Read the model definition and answer for the solid it produces. Units are mm, in the model's axes. A direction names the side the tool comes from. Coordinates: 2 decimals unless noted, no trailing zeros. Write each loop counter-clockwise with the first axis right and the second up, starting at its lowest first coordinate (ties: lowest second). Pieces come first, ordered by that corner, then holes.
Item 1: Straight lines are drawn through the part: probe 1 along X at (y, z) = (-6, -6.5); probe 2 along Z at (x, y) = (8.5, 3); probe 3 along X at (y, z) = (-8, -4). For each, find the intervals that lie inside material, in ascending order.
Item 2: Section A-A (z = -1.75) is taken. Give the vertices of the cut face in (x, y), then the cut area to 3 significant figures.
Item 3: Section B-B (x = 24.5) is taken. Give the vertices of the cut face in (y, z), then the cut area to 3 significant figures.
Item 4: Each of these flat-tipped pins is pushed along its axis until it touches: P1, Ø1, axis at y = 1.5, z = -5, coming from the -X side; P2, Ø1.5, axis at x = 15, y = 3, coming from the -Z side; P3, Ø2, axis at y = -1.5, z = -6, coming from the -X side. Where does it stop, or does it pass through?
Item 5: A tool of negligible diameter and unlimited length cuts with its end or side. For faces 4 (the face through (53, 9, 0)), 5 (the face through (84.524, 2.772, 5.986)), 6 (the face through (107, 0, -6)), from which of +Z, -Z, +X, -X, +Y, -Y can it reach the whole face along a straight path? Write none if from no direction.
Item 6: Determine the mould class of faces 1 (the face through (33, -9, 0)), 2 (the face through (84.108, 0.815, -0.098)), 3 (the face through (-9, 0, 0)) for opening direction X: released by +X, released by -X, zero draft, split by the parting line, or undercut.
Item 7: Section C-C (x = 81) is taken. Give the vertices of the cut face in (y, z).
from build123d import *
from build123d.topology import SkipClean

# Parameters (mm, degrees)
BOSS_EXTRUDE1_DEPTH = 5
BOSS_EXTRUDE2_START = -12
BOSS_EXTRUDE2_DEPTH = 14


with BuildPart() as part:
    # Sketch1 → Boss-Extrude1 (new, symmetric)
    with SkipClean():  # the faces are left unmerged after this step: merging them gives an invalid solid
        with BuildSketch(Plane.XY):
            with BuildLine():
                ThreePointArc((9, 0), (6.363961031, -6.363961031), (0, -9))
                Line((0, -9), (66.272706331, -9))
                ThreePointArc((66.272706331, -9), (68.43776984, -7.75), (68.43776984, -5.25))
                ThreePointArc((68.43776984, -5.25), (67.583242863, 0.670186682), (73.015870906, 3.173260641))
                Line((73.015870906, 3.173260641), (95.515870906, -1.609261996))
                ThreePointArc((95.515870906, -1.609261996), (97.934586459, -2.888858783), (99.317541634, -5.25))
                ThreePointArc((99.317541634, -5.25), (104.158770817, -9), (109, -5.25))
                Line((109, -5.25), (109, 5))
                ThreePointArc((109, 5), (107.828427125, 7.828427125), (105, 9))
                Line((105, 9), (0, 9))
                ThreePointArc((0, 9), (6.363961031, 6.363961031), (9, 0))
            make_face()
            with BuildLine():
                ThreePointArc((-9, 0), (-6.363961031, -6.363961031), (0, -9))
                ThreePointArc((0, -9), (6.363961031, -6.363961031), (9, 0))
                Line((9, 0), (4.75, 0))
                ThreePointArc((4.75, 0), (0, -4.75), (-4.75, 0))
                Line((-4.75, 0), (-9, 0))
            make_face()
            with BuildLine():
                ThreePointArc((0, 9), (-6.363961031, 6.363961031), (-9, 0))
                Line((-9, 0), (-4.75, 0))
                ThreePointArc((-4.75, 0), (0, 4.75), (4.75, 0))
                Line((4.75, 0), (9, 0))
                ThreePointArc((9, 0), (6.363961031, 6.363961031), (0, 9))
            make_face()
            with BuildLine():
                ThreePointArc((-9, 0), (-6.363961031, -6.363961031), (0, -9))
                ThreePointArc((0, -9), (6.363961031, -6.363961031), (9, 0))
                Line((9, 0), (4.75, 0))
                ThreePointArc((4.75, 0), (0, -4.75), (-4.75, 0))
                Line((-4.75, 0), (-9, 0))
            make_face()
            with BuildLine():
                ThreePointArc((0, 9), (-6.363961031, 6.363961031), (-9, 0))
                Line((-9, 0), (-4.75, 0))
                ThreePointArc((-4.75, 0), (0, 4.75), (4.75, 0))
                Line((4.75, 0), (9, 0))
                ThreePointArc((9, 0), (6.363961031, 6.363961031), (0, 9))
            make_face()
        extrude(amount=BOSS_EXTRUDE1_DEPTH, both=True)

    # Sketch2 → Boss-Extrude2 (add)
    with SkipClean():  # the faces are left unmerged after this step: merging them gives an invalid solid
        with BuildSketch(Plane.XY.offset(5).offset(BOSS_EXTRUDE2_START)):
            with BuildLine():
                Line((105, 9), (0, 9))
                ThreePointArc((0, 9), (-9, 0), (0, -9))
                Line((0, -9), (66.272706331, -9))
                ThreePointArc((66.272706331, -9), (68.43776984, -7.75), (68.43776984, -5.25))
                ThreePointArc((68.43776984, -5.25), (67.583242863, 0.670186682), (73.015870906, 3.173260641))
                Line((73.015870906, 3.173260641), (95.515870906, -1.609261996))
                ThreePointArc((95.515870906, -1.609261996), (97.934586459, -2.888858783), (99.317541634, -5.25))
                ThreePointArc((99.317541634, -5.25), (104.158770817, -9), (109, -5.25))
                Line((109, -5.25), (109, 5))
                ThreePointArc((109, 5), (107.828427125, 7.828427125), (105, 9))
            make_face()
            with BuildLine():
                Line((105, 7), (0, 7))
                ThreePointArc((0, 7), (-7, 0), (0, -7))
                Line((0, -7), (66.272706331, -7))
                ThreePointArc((66.272706331, -7), (66.664953896, -6.810067489), (66.7591992, -6.38456739))
                ThreePointArc((66.7591992, -6.38456739), (65.919794123, 1.792306924), (73.431694287, 5.129555843))
                Line((73.431694287, 5.129555843), (95.931694287, 0.347033205))
                ThreePointArc((95.931694287, 0.347033205), (99.317896062, -1.444402296), (101.254033308, -4.75))
                ThreePointArc((101.254033308, -4.75), (104.047625793, -6.997940424), (107, -4.963024782))
                Line((107, -4.963024782), (107, 5))
                ThreePointArc((107, 5), (106.414213562, 6.414213562), (105, 7))
            make_face(mode=Mode.SUBTRACT)
        extrude(amount=BOSS_EXTRUDE2_DEPTH)


solid = part.part
Established:
1. probe 1: x = -6.71 to -3.61, 66.44 to 68.72, 99.58 to 101.92, 106.39 to 108.74
1. probe 2: z = -5 to 5
1. probe 3: x = -4.12 to 68.27, 101.16 to 107.16
2. outline: (0, -9) - (66.27, -9) arc R2.5 ccw to (68.44, -5.25) arc R5 cw to (73.02, 3.17) - (95.52, -1.61) arc R5 cw to (99.32, -5.25) arc R5 ccw to (109, -5.25) - (109, 5) arc R4 ccw to (105, 9) - (0, 9) arc R9 ccw to start; hole circle Ø9.5 at (0, 0)
2. area: 1,700 mm2
3. outline: (-9, -7) - (-7, -7) - (-7, -5) - (7, -5) - (7, -7) - (9, -7) - (9, 7) - (7, 7) - (7, 5) - (-7, 5) - (-7, 7) - (-9, 7) - close
3. area: 196 mm2
4. P1: stops at x = -8.94
4. P2: stops at z = -5
4. P3: stops at x = -8.99
5. face 4: +Z, -Z, +X, -X, +Y
5. face 5: +Z
5. face 6: -Z
6. face 1: zero draft
6. face 2: undercut
6. face 3: released by -X
7. outline: (1.48, -7) - (3.52, -7) - (3.52, -5) - (7, -5) - (7, -7) - (9, -7) - (9, 7) - (7, 7) - (7, 5) - (3.52, 5) - (3.52, 7) - (1.48, 7) - close
